```python
from build123d import *

# Parameters (mm, degrees)
SKETCH1_W                       = 12
SKETCH1_H                       = 14
SKETCH1_R                       = 1.2
BOSS_EXTRUDE1_DEPTH             = 3
SKETCH3_R                       = 3
BOSS_EXTRUDE2_DEPTH             = 6
BOSS_EXTRUDE2_DIRECTION_2_REACH = 11.695
FILLET1_R                       = 2
BOSS_EXTRUDE3_DEPTH             = 3
SKETCH6_R                       = 2.1
CUT_EXTRUDE2_DEPTH              = 1
SKETCH10_R                      = 1.5
CUT_EXTRUDE3_DEPTH              = 6
CHAMFER1_SIZE                   = 0.6


with BuildPart() as part:
    # Sketch1 → Boss-Extrude1 (new body)
    with BuildSketch(Plane(origin=(0, 0, 0), x_dir=(1, 0, 0), z_dir=(0, 1, 0))):
        Rectangle(SKETCH1_W, SKETCH1_H)
        with Locations(Location((0, 4, 0), (0, 0, 270))):
            Circle(SKETCH1_R, mode=Mode.SUBTRACT)
        with Locations(Location((0, -4, 0), (0, 0, 270))):
            Circle(SKETCH1_R, mode=Mode.SUBTRACT)
    extrude(amount=BOSS_EXTRUDE1_DEPTH)

    # Sketch3 → Boss-Extrude2 (add)
    with BuildSketch(Plane(origin=(0, 3, 0), x_dir=(1, 0, 0), z_dir=(0, 1, 0))):
        with Locations(Location((-6, 0, 0), (0, 0, 270))):
            Circle(SKETCH3_R)
    extrude(amount=BOSS_EXTRUDE2_DEPTH)

    # Boss-Extrude2 direction 2: up to this face of the body (flat: up to its plane)
    boss_extrude2_direction_2_end = Plane(part.part.faces().sort_by_distance((0, 0, 0))[0])
    # Sketch3 → Boss-Extrude2 direction 2 (add, up to the picked face)
    with BuildSketch(Plane(origin=(0, 3, 0), x_dir=(1, 0, 0), z_dir=(0, 1, 0)), mode=Mode.PRIVATE) as boss_extrude2_direction_2_sk1:
        with Locations(Location((-6, 0, 0), (0, 0, 270))):
            Circle(SKETCH3_R)
    boss_extrude2_direction_2_tool1 = split(extrude(boss_extrude2_direction_2_sk1.sketch, amount=-BOSS_EXTRUDE2_DIRECTION_2_REACH, mode=Mode.PRIVATE), bisect_by=boss_extrude2_direction_2_end, keep=Keep.BOTH, mode=Mode.PRIVATE)
    add(boss_extrude2_direction_2_tool1.solids().sort_by(Axis((-6, 3, 0), (0, -1, 0)))[0])

    # Fillet1
    fillet1_edges = [part.edges().sort_by_distance(p)[0] for p in [
        (6, 1.5, 7),
        (-6, 1.5, 7),
        (-6, 1.5, -7),
        (6, 1.5, -7),
    ]]
    fillet(fillet1_edges, radius=FILLET1_R)

    # Sketch5 → Boss-Extrude3 (add)
    with BuildSketch(Plane(origin=(0, 3, 0), x_dir=(1, 0, 0), z_dir=(0, 1, 0))):
        with BuildLine():
            Line((-8.530087563, 1.612035025), (-5.686725042, 6.074690017))
            ThreePointArc((-5.686725042, 6.074690017), (-5.920084645, 5.559709709), (-6, 5))
            Line((-6, 5), (-6, 3))
            ThreePointArc((-6, 3), (-7.442895513, 2.630219105), (-8.530087563, 1.612035025))
        make_face()
        with BuildLine():
            Line((-8.530087563, -1.612035025), (-5.686725042, -6.074690017))
            ThreePointArc((-5.686725042, -6.074690017), (-5.920084645, -5.559709709), (-6, -5))
            Line((-6, -5), (-6, -3))
            ThreePointArc((-6, -3), (-7.442895513, -2.630219105), (-8.530087563, -1.612035025))
        make_face()
    extrude(amount=-BOSS_EXTRUDE3_DEPTH)

    # Sketch6 → Cut-Extrude2 (cut)
    with BuildSketch(Plane(origin=(0, 3, 0), x_dir=(1, 0, 0), z_dir=(0, 1, 0))):
        with Locations(Location((0, 4, 0), (0, 0, 270))):
            Circle(SKETCH6_R)
        with Locations(Location((0, -4, 0), (0, 0, 270))):
            Circle(SKETCH6_R)
    extrude(amount=-CUT_EXTRUDE2_DEPTH, mode=Mode.SUBTRACT)

    # Sketch10 → Cut-Extrude3 (cut)
    with BuildSketch(Plane(origin=(0, 9, 0), x_dir=(1, 0, 0), z_dir=(0, 1, 0))):
        with Locations(Location((-6, 0, 0), (0, 0, 270))):
            Circle(SKETCH10_R)
    extrude(amount=-CUT_EXTRUDE3_DEPTH, mode=Mode.SUBTRACT)

    # Chamfer1
    chamfer1_edges = [part.edges().sort_by_distance(p)[0] for p in [
        (-6, 9, -1.5),
    ]]
    chamfer(chamfer1_edges, length=CHAMFER1_SIZE)


solid = part.part
```
Check sheet for the modelled part. Datum: model origin and axes. Units: mm. A direction names the side the tool comes from. Give positions to 0.01 mm unless a question says otherwise; leave off trailing zeros. Order: outer loops, then holes, each group sorted by start corner. A loop starts at its lowest first (then second) coordinate and runs counter-clockwise, first axis right, second up. Notation, with made-up numbers: (29, -12.75) -> (81, -12.75) arc R5 cw to (81, -5.75) -> close; hole circle Ø11 at (66, 55.25). An arc over 180 degrees is marked (long way). Use CSV: the item, a comma, the result in double quotes. Start each with the question number.
1) Go/stop test with flat-tipped pins: P1, Ø3, axis at x = 0, z = 4, coming from the -Y side; P2, Ø0.9, axis at x = -6, z = 0, coming from the +Y side; P3, Ø1, axis at y = 5, z = -4.5, coming from the -X side; P4, Ø2, axis at x = -1, z = -4, coming from the +Y side. Record where each tip stops, or that it passes through.
2) Sectioned sample at C-C, the plane y = 2.75. Record the boundary of the cut face in (x, z).
3) Sectioned sample at D-D, the plane y = 7.75. Record the boundary of the cut face in (x, z), plus the area to 3 significant figures.
4) Sectioned sample at A-A, the plane x = 0. Record the boundary of the cut face in (y, z), plus the area to 3 significant figures.
5) Mould release check, pull along X, two halves, no side actions. Record for faces 1 (the face through (0.631, 2.507, 6.003)), 2 (the face through (-4.97, 1.52, 6.75)), 3 (the face through (-2, 0, 0)), 4 (the face through (1.01, 0.99, 4.65)): released by +X, released by -X, zero draft, split by the parting line, or undercut.
6) Set-up check for faces 5 (the face through (-6, 3, 0)), 6 (the face through (-7.13, 1.52, 3.81)): record each of +Z, -Z, +X, -X, +Y, -Y from which the full face is reachable in a straight line by a thin tool's end or side.
7) Sectioned sample at B-B, the plane z = -4.25. Record the boundary of the cut face in (x, y), plus the area to 3 significant figures.
8) Material ranges on line 1 (Z direction, x = -0.25, y = 0.5); line 2 (Y direction, x = -4.5, z = -6); line 3 (X direction, y = 0.8, z = -4), recorded low to high. Write a range as from..to.
Recorded:
1,P1,"y = 0"
1,P2,"y = 3"
1,P3,"through"
1,P4,"y = 2"
2,outline,"(-8.53, -1.61) -> (-5.69, -6.07) arc R2 ccw to (-4, -7) -> (4, -7) arc R2 ccw to (6, -5) -> (6, 5) arc R2 ccw to (4, 7) -> (-4, 7) arc R2 ccw to (-5.69, 6.07) -> (-8.53, 1.61) arc R3 ccw to start; hole circle Ø4.2 at (0, -4); hole circle Ø4.2 at (0, 4)"
3,outline,"circle Ø6 at (-6, 0); hole circle Ø3 at (-6, 0)"
3,area,"21.2 mm2"
4,outline,"(0, -7) -> (3, -7) -> (3, -6.1) -> (2, -6.1) -> (2, -5.2) -> (0, -5.2) -> close; (0, -2.8) -> (2, -2.8) -> (2, -1.9) -> (3, -1.9) -> (3, 1.9) -> (2, 1.9) -> (2, 2.8) -> (0, 2.8) -> close; (0, 5.2) -> (2, 5.2) -> (2, 6.1) -> (3, 6.1) -> (3, 7) -> (0, 7) -> close"
4,area,"24.0 mm2"
5,face 1,"undercut"
5,face 2,"released by -X"
5,face 3,"zero draft"
5,face 4,"undercut"
6,face 5,"+Y"
6,face 6,"+Z, -X, +Y, -Y"
7,outline,"(-6.85, 0) -> (-1.17, 0) -> (-1.17, 2) -> (-2.09, 2) -> (-2.09, 3) -> (-6.85, 3) -> close; (1.17, 0) -> (6, 0) -> (6, 3) -> (2.09, 3) -> (2.09, 2) -> (1.17, 2) -> close"
7,area,"29.7 mm2"
8,line 1,"-7..-5.17, -2.83..2.83, 5.17..7"
8,line 2,"0..3"
8,line 3,"-7.01..-1.2, 1.2..6"
